Geometry check sheet. Reference: the model listing, model coordinates, mm. Coordinates: 2 decimals unless noted, no trailing zeros. Write each loop counter-clockwise with the first axis right and the second up, starting at its lowest first coordinate (ties: lowest second). Pieces come first, ordered by that corner, then holes. Notation, with made-up numbers: (-18, -11) -> (23, -11) arc R27 ccw to (23, 5) -> close; hole circle Ø1 at (-8, -3). An arc over 180 degrees is marked (long way). Answer in a Markdown table with one row per item. Add a question column.
Q1. Gauge pin test, flat ends, axial feed: P1, Ø10, axis at x = 8.5, y = -11, coming from the +Z side; P2, Ø12, axis at x = -4, z = -19.5, coming from the -Y side; P3, Ø12, axis at x = 14.5, z = -6.5, coming from the +Y side; P4, Ø8, axis at y = -8, z = -6, coming from the -X side. Record the tip position at first contact, or that the pin passes through.
Q2. Release check for a two-part mould opening along X. For faces 1 (the face through (0, 0, 0)), 2 (the face through (-0.59, -4.46, -19.34)), 3 (the face through (0.267, -2.033, -20.86)) record: pulls with the +X half, pulls with the -X half, needs draft (parallel to the pull), parting line crosses it, or undercut.
Q3. Section check C-C, the plane z = -18.5. Record the boundary of the cut face in (x, y).
Q4. Section check B-B, the plane y = 3. Record the boundary of the cut face in (x, z), and give its area (3 significant figures).
Q5. Section check D-D, the plane x = 6. Record the boundary of the cut face in (y, z).
Q6. Section check A-A, the plane z = -6. Record the boundary of the cut face in (x, y).
Q7. Thickness scan on line 1 (Y direction, x = 0, z = -19); line 2 (Z direction, x = -8.5, y = 1); line 3 (Y direction, x = -0.5, z = -3). Record the ranges inside material, lowest first.
```python
from build123d import *

# Parameters (mm, degrees)
F0_R     = 20
F1_DEPTH = 8
F2_R     = 4.5
F3_DEPTH = 23
F5_D     = 4.1
F5_DEPTH = 20
F5_TIP   = 1.231764269


with BuildPart() as f1:
    # F0 (on Top) → F1 (new body)
    with BuildSketch(Plane.XY):
        Circle(F0_R)
    extrude(amount=-F1_DEPTH)

    # F2 (on face) → F3 (join)
    with BuildSketch(Plane(origin=(0, 0, -8), x_dir=(1, 0, 0), z_dir=(0, 0, -1))):
        Circle(F2_R)
    extrude(amount=F3_DEPTH)

    # F5
    with Locations(Plane(origin=(0, 0, -31), x_dir=(1, 0, 0), z_dir=(0, 0, -1))):
        with Locations((0, 0)):
            Hole(F5_D / 2, depth=F5_DEPTH)
            with Locations((0, 0, -(F5_DEPTH + F5_TIP / 2))):  # 118° drill point
                Cone(0, F5_D / 2, F5_TIP, mode=Mode.SUBTRACT)


solid = f1.part
```
Calculated:
| question | item | result |
|---|---|---|
| 1 | P1 | stops at z = 0 |
| 1 | P2 | stops at y = -4.5 |
| 1 | P3 | stops at y = 18.1 |
| 1 | P4 | stops at x = -19.6 |
| 2 | face 1 | needs draft |
| 2 | face 2 | parting line crosses it |
| 2 | face 3 | undercut |
| 3 | outline | circle Ø9 at (0, 0); hole circle Ø4.1 at (0, 0) |
| 4 | outline | (-19.77, -8) -> (-3.35, -8) -> (-3.35, -31) -> (3.35, -31) -> (3.35, -8) -> (19.77, -8) -> (19.77, 0) -> (-19.77, 0) -> close |
| 4 | area | 471 mm² |
| 5 | outline | (-19.08, -8) -> (19.08, -8) -> (19.08, 0) -> (-19.08, 0) -> close |
| 6 | outline | circle Ø40 at (0, 0) |
| 7 | line 1 | y = -4.5 to -2.05, 2.05 to 4.5 |
| 7 | line 2 | z = -8 to 0 |
| 7 | line 3 | y = -19.99 to 19.99 |
